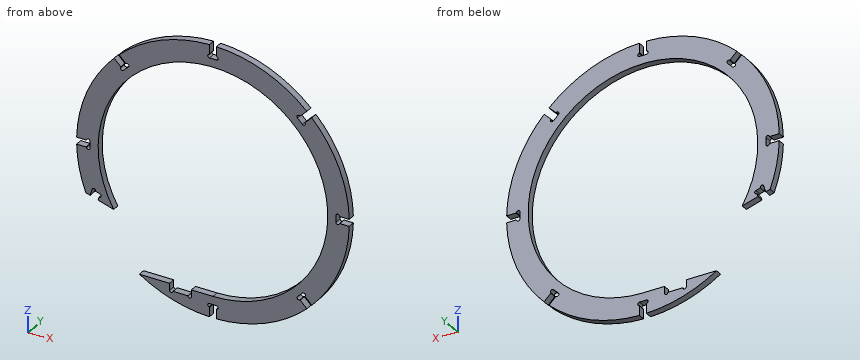
from build123d import *

# Parameters (mm, degrees)
SKETCH1_R                = 250
SKETCH1_R_2              = 210.5
BOSS_EXTRUDE1_DEPTH      = 12.7
CUT_EXTRUDE1_DEPTH       = 354.781415566
FILLET1_R                = 1
CIRPATTERN1_COUNT        = 8
FILLET1_OF_CIRPATTERN1_R = 1
CUT_EXTRUDE3_DEPTH       = 354.665618911
CUT_EXTRUDE4_DEPTH       = 354.665618911


with BuildPart() as part:
    # Sketch1 → Boss-Extrude1 (new body)
    with BuildSketch(Plane(origin=(0, 0, 0), x_dir=(1, 0, 0), z_dir=(0, 1, 0))):
        with Locations(Location((0, 0, 0), (0, 0, 270))):
            Circle(SKETCH1_R)
        with Locations(Location((0, 0, 0), (0, 0, 270))):
            Circle(SKETCH1_R_2, mode=Mode.SUBTRACT)
    extrude(amount=BOSS_EXTRUDE1_DEPTH)

    # Sketch2 → Cut-Extrude1 (cut, through all)
    with BuildSketch(Plane(origin=(0, 12.7, 0), x_dir=(1, 0, 0), z_dir=(0, 1, 0))):
        with BuildLine():
            Line((6.4, 225.5), (-6.4, 225.5))
            ThreePointArc((-6.4, 225.5), (-9.6, 228.7), (-6.4, 231.9))
            Line((-6.4, 231.9), (-6.4, 250))
            Line((-6.4, 250), (6.4, 250))
            Line((6.4, 250), (6.4, 231.9))
            ThreePointArc((6.4, 231.9), (9.6, 228.7), (6.4, 225.5))
        make_face()
    cut_extrude1 = extrude(amount=-CUT_EXTRUDE1_DEPTH, mode=Mode.SUBTRACT)

    # Fillet1
    fillet1_edges = [part.edges().sort_by_distance(p)[0] for p in [
        (-6.4, 6.35, -231.9),
        (6.4, 6.35, -231.9),
    ]]
    fillet(fillet1_edges, radius=FILLET1_R)

    # CirPattern1: Cut-Extrude1 ×8 about axis
    cirpattern1_axis = Axis((0, 0, 0), (0, 1, 0))
    for i in range(1, CIRPATTERN1_COUNT):
        add(cut_extrude1.rotate(cirpattern1_axis, i * 360 / CIRPATTERN1_COUNT), mode=Mode.SUBTRACT)

    # Fillet1 of CirPattern1
    fillet1_of_cirpattern1_edges = [part.edges().sort_by_distance(p)[0] for p in [
        (-168.503545957, 6.35, -159.452579158),
        (-159.452579158, 6.35, -168.503545957),
        (-231.9, 6.35, 6.4),
        (-231.9, 6.35, -6.4),
        (-159.452579158, 6.35, 168.503545957),
        (-168.503545957, 6.35, 159.452579158),
        (6.4, 6.35, 231.9),
        (-6.4, 6.35, 231.9),
        (168.503545957, 6.35, 159.452579158),
        (159.452579158, 6.35, 168.503545957),
        (231.9, 6.35, -6.4),
        (231.9, 6.35, 6.4),
        (159.452579158, 6.35, -168.503545957),
        (168.503545957, 6.35, -159.452579158),
    ]]
    fillet(fillet1_of_cirpattern1_edges, radius=FILLET1_OF_CIRPATTERN1_R)

    # Sketch5 → Cut-Extrude3 (cut, through all)
    with BuildSketch(Plane(origin=(0, 12.7, 0), x_dir=(1, 0, 0), z_dir=(0, 1, 0))):
        Polygon((0, 210.5), (-248.044523643, 210.5), (-248.044523643, 90.5), (-233.044523643, 90.5), (0, 160.5), align=None)
    extrude(amount=-CUT_EXTRUDE3_DEPTH, mode=Mode.SUBTRACT)

    # Sketch6 → Cut-Extrude4 (cut, through all)
    with BuildSketch(Plane(origin=(0, 12.7, 0), x_dir=(1, 0, 0), z_dir=(0, 1, 0))):
        with BuildLine():
            Line((-39.506660352, 210.5), (-39.506660352, 223.2))
            ThreePointArc((-39.506660352, 223.2), (-42.706660352, 226.4), (-45.906660352, 223.2))
            Line((-45.906660352, 223.2), (-73.106660352, 223.2))
            ThreePointArc((-73.106660352, 223.2), (-76.306660352, 226.4), (-79.506660352, 223.2))
            Line((-79.506660352, 223.2), (-79.506660352, 210.5))
            Line((-79.506660352, 210.5), (-39.506660352, 210.5))
        make_face()
        with BuildLine():
            Line((-225.095552296, 92.887646728), (-221.442085646, 80.724498227))
            ThreePointArc((-221.442085646, 80.724498227), (-217.45679679, 78.580326423), (-215.312624985, 82.565615279))
            Line((-215.312624985, 82.565615279), (-207.076162221, 85.039616318))
            ThreePointArc((-207.076162221, 85.039616318), (-204.931990416, 89.024905174), (-208.917279273, 91.169076979))
            Line((-208.917279273, 91.169076979), (-210.72962887, 97.202764818))
            Line((-210.72962887, 97.202764818), (-225.095552296, 92.887646728))
        make_face()
    extrude(amount=-CUT_EXTRUDE4_DEPTH, mode=Mode.SUBTRACT)


solid = part.part
Verification items for the finished model (mm, model axes). Give positions to 0.01 mm unless a question says otherwise; leave off trailing zeros. Write each loop counter-clockwise with the first axis right and the second up, starting at its lowest first coordinate (ties: lowest second). Pieces come first, ordered by that corner, then holes.
(1) Cross-section at A-A (z = 0). Enter the section's corners in (x, y).
(2) Gauge pin test, flat ends, axial feed: pin 1 (6.5 mm diameter, centred on x = -100.5, y = 4.5, fed in from +Z); pin 2 (4 mm diameter, centred on y = 9, z = -94, fed in from +X); pin 3 (2 mm diameter, centred on x = 103.5, y = 11, fed in from +Z). Record the tip position at first contact, or that the pin passes through.
(3) Cross-section at B-B (x = 36.5). Enter the section's corners in (y, z), plus the area to 3 significant figures.
(4) Material ranges on line 1 (Z direction, x = 0, y = 3.5); line 2 (X direction, y = 1, z = -81), recorded low to high.
Worked out:
1. outline: (-225.5, 0) - (-210.5, 0) - (-210.5, 12.7) - (-225.5, 12.7) - close; (210.5, 0) - (225.5, 0) - (225.5, 12.7) - (210.5, 12.7) - close
2. pin 1: stops at z = 230.31
2. pin 2: stops at x = 232.46
2. pin 3: stops at z = 228.02
3. outline: (0, -247.32) - (12.7, -247.32) - (12.7, -207.31) - (0, -207.31) - close; (0, 207.31) - (12.7, 207.31) - (12.7, 247.32) - (0, 247.32) - close
3. area: 1,020 mm2
4. line 1: z = -225.5 to -210.5, 210.5 to 225.5
4. line 2: x = -236.51 to -221.52, -215.24 to -194.29, 194.29 to 236.51
